from build123d import *

# Parameters (mm, degrees)
SKETCH_1_W                  = 10
SKETCH_1_H                  = 20
SKETCH_1_W_2                = 8
SKETCH_1_H_2                = 25
EXTRUDE_1_DEPTH             = 8
HOLE_WIZARD_M4_1_AT_2_COUNT = 2
HOLE_WIZARD_M4_1_AT_2_PITCH = 34
HOLE_WIZARD_M4_1_2_D        = 4.5
HOLE_WIZARD_M4_1_2_DEPTH    = 8
SKETCH_7_R                  = 2.25
CUT_EXTRUDE_1_DEPTH         = 4


with BuildPart() as part:
    # 스케치1 → 보스-돌출1 (new body)
    with BuildSketch(Plane(origin=(0, 0, 0), x_dir=(1, 0, 0), z_dir=(0, 1, 0))):
        with Locations((0, 22.5)):
            Rectangle(SKETCH_1_W, SKETCH_1_H)
        Rectangle(SKETCH_1_W_2, SKETCH_1_H_2)
        with Locations((0, -22.5)):
            Rectangle(SKETCH_1_W, SKETCH_1_H)
    extrude(amount=EXTRUDE_1_DEPTH)

    # 스케치3 → Hole Wizard M4 _ _ _ _ _ _1 (revolve, cut)
    with BuildSketch(Plane(origin=(0, 8, -17), x_dir=(0, 0, 1), z_dir=(1, 0, 0))):
        Polygon((0, 0), (0, 8), (2.25, 8), (2.25, 4.4), (4, 4.4), (4, 0.7), (4.7, 0), align=None)
    hole_wizard_m4_1 = revolve(axis=Axis((0, 14.35, -17), (0, -1, 0)), mode=Mode.SUBTRACT)

    # Hole Wizard M4 _ _ _ _ _ _1 at 2: Hole Wizard M4 _ _ _ _ _ _1 ×2
    with Locations(*[(0, 0, i * HOLE_WIZARD_M4_1_AT_2_PITCH) for i in range(1, HOLE_WIZARD_M4_1_AT_2_COUNT)]):
        add(hole_wizard_m4_1, mode=Mode.SUBTRACT)

    # Hole Wizard M4 _ _1 2
    with Locations(Plane(origin=(0, 0, 0), x_dir=(-1, 0, 0), z_dir=(0, -1, 0))):
        with Locations((0, -27.5), (0, 27.5), (54.10839937, -109.42081154)):
            Hole(HOLE_WIZARD_M4_1_2_D / 2, depth=HOLE_WIZARD_M4_1_2_DEPTH)

    # 스케치7 → 컷-돌출1 (cut)
    with BuildSketch(Plane.XZ):
        Polygon((2.049593456, -31.05), (4.099186911, -27.5), (2.049593456, -23.95), (-2.049593456, -23.95), (-4.099186911, -27.5), (-2.049593456, -31.05), align=None)
        with Locations((0, -27.5)):
            Circle(SKETCH_7_R, mode=Mode.SUBTRACT)
        Polygon((2.049593456, 23.95), (-2.049593456, 23.95), (-4.099186911, 27.5), (-2.049593456, 31.05), (2.049593456, 31.05), (4.099186911, 27.5), align=None)
        with Locations((0, 27.5)):
            Circle(SKETCH_7_R, mode=Mode.SUBTRACT)
    extrude(amount=-CUT_EXTRUDE_1_DEPTH, mode=Mode.SUBTRACT)


solid = part.part
Input: part model. Units: mm. Frame: model coordinates. A direction names the side the tool comes from. Give positions to 0.01 mm unless a question says otherwise; leave off trailing zeros. Write each loop counter-clockwise with the first axis right and the second up, starting at its lowest first coordinate (ties: lowest second). Pieces come first, ordered by that corner, then holes. Notation, with made-up numbers: (78, -5.5) -> (126, -5.5) arc R23 ccw to (126, 26.5) -> close; hole circle Ø9 at (9.25, 53.5). An arc over 180 degrees is marked (long way). Use one line per item in the form item = value. Start each with the question number.
1) Pin query (flat end, axial travel): pin 1 (2.5 mm diameter, centred on x = 0, z = 17, fed in from +Y); pin 2 (3.5 mm diameter, centred on x = 1, z = -27.5, fed in from -Y); pin 3 (4 mm diameter, centred on y = 6, z = -3.5, fed in from -X); pin 4 (4 mm diameter, centred on y = 2, z = -3, fed in from +X). Return the tip coordinate at first contact, or that it passes through.
2) Section query C-C on y = 2. Return the cut outline in (x, z).
3) Section query B-B on y = 5.75. Return the cut outline in (x, z), then the cut area to 3 significant figures.
4) Set-up query: faces 3 (the cylindrical face through (-0.488, 6.028, -25.304)), 4 (the flat face through (3.09, 1.97, 25.75)), 5 (the flat face through (-4.5, 3.9, 12.5)), 6 (the flat face through (4.5, 3.9, -12.5)). Return all of +Z, -Z, +X, -X, +Y, -Y with unobstructed straight access to the full face (end or side cutting, diameter ignored); none if empty.
5) Ray query, probe 1 along Z at (x, y) = (0, 6.55); probe 2 along Z at (x, y) = (0, 2.2); probe 3 along X at (y, z) = (4.95, 17). Return the intervals inside material, ascending. Write a range as from..to.
6) Section query A-A on z = 17. Return the cut outline in (x, y).
7) Draft query along Z for faces 1 (the cylindrical face through (0.86, 1.83, 19.08)), 2 (the flat face through (0, 0, 0)). Return one class per face: pulls with the +Z half, pulls with the -Z half, needs draft (parallel to the pull), parting line crosses it, or undercut.
8) Section query D-D on x = 0. Count the separate pieces of the cut face and the enclosed holes in it, then the cut area to 3 significant figures.
Outcome:
q1.pin_1 = through
q1.pin_2 = 4
q1.pin_3 = -4
q1.pin_4 = 4
q2.outline = (-5, -32.5) -> (5, -32.5) -> (5, -12.5) -> (4, -12.5) -> (4, 12.5) -> (5, 12.5) -> (5, 32.5) -> (-5, 32.5) -> (-5, 12.5) -> (-4, 12.5) -> (-4, -12.5) -> (-5, -12.5) -> close; hole (-4.1, -27.5) -> (-2.05, -31.05) -> (2.05, -31.05) -> (4.1, -27.5) -> (2.05, -23.95) -> (-2.05, -23.95) -> close; hole (-4.1, 27.5) -> (-2.05, 23.95) -> (2.05, 23.95) -> (4.1, 27.5) -> (2.05, 31.05) -> (-2.05, 31.05) -> close; hole circle Ø4.5 at (0, -17); hole circle Ø4.5 at (0, 17)
q3.outline = (-5, -32.5) -> (5, -32.5) -> (5, -12.5) -> (4, -12.5) -> (4, 12.5) -> (5, 12.5) -> (5, 32.5) -> (-5, 32.5) -> (-5, 12.5) -> (-4, 12.5) -> (-4, -12.5) -> (-5, -12.5) -> close; hole circle Ø8 at (0, -17); hole circle Ø8 at (0, 17); hole circle Ø4.5 at (0, -27.5); hole circle Ø4.5 at (0, 27.5)
q3.area = 468 mm^2
q4.face_3 = +Y, -Y
q4.face_4 = -Y
q4.face_5 = -X, +Y, -Y
q4.face_6 = +X, +Y, -Y
q5.probe_1 = -32.5..-29.75, -25.25..-21, -13..13, 21..25.25, 29.75..32.5
q5.probe_2 = -32.5..-31.05, -23.95..-19.25, -14.75..14.75, 19.25..23.95, 31.05..32.5
q5.probe_3 = -5..-4, 4..5
q6.outline = (-5, 0) -> (-2.25, 0) -> (-2.25, 3.6) -> (-4, 3.6) -> (-4, 7.3) -> (-4.7, 8) -> (-5, 8) -> close; (2.25, 0) -> (5, 0) -> (5, 8) -> (4.7, 8) -> (4, 7.3) -> (4, 3.6) -> (2.25, 3.6) -> close
q7.face_1 = undercut
q7.face_2 = needs draft
q8.separate_pieces = 5
q8.enclosed_holes = 0
q8.area = 323 mm^2
